Design review of the part built by this model. Coordinates are the model's own, in mm. Face numbers are marked on the shaded views. A direction names the side the tool comes from. Coordinates: 2 decimals unless noted, no trailing zeros. Write each loop counter-clockwise with the first axis right and the second up, starting at its lowest first coordinate (ties: lowest second). Pieces come first, ordered by that corner, then holes. Notation, with made-up numbers: (-4.5, 16.5) -> (27.5, 16.5) arc R18 cw to (27.5, 48.5) -> close; hole circle Ø5 at (38, -36). An arc over 180 degrees is marked (long way). One line per question, with ' | ' between items. Start each with the question number.
Q1. Add section C-C on y = -45.5. State the section outline as (x, z) points, and give its area (3 significant figures).
Q2. For P1, Ø2, axis at x = -4, z = -21.5, coming from the -Y side; P2, Ø4, axis at x = -4, y = -69.5, coming from the +Z side; P3, Ø3, axis at x = 0, y = -31.75, coming from the +Z side; P4, Ø2, axis at x = 3, z = -7.5, coming from the +Y side, all flat-tipped, find the tip position at first contact; note any pin that passes through.
Q3. Add section B-B on x = 0. Give the number of separate pieces and of enclosed holes in the cut face, and give its area (3 significant figures).
Q4. Wall thickness on probe 1 along Z at (x, y) = (3.25, -50.5); probe 2 along Z at (x, y) = (-5.5, -60.5); probe 3 along Y at (x, z) = (-0.5, -16.5): over which ranges is each line inside the solid? List them lowest first.
Q5. Add section A-A on y = -15. State the section outline as (x, z) points.
Q6. Add section D-D on y = -57.5. State the section outline as (x, z) points, and give its area (3 significant figures).
Q7. For the marked faces 5 and 6, list the 3-axis set-ups (+Z, -Z, +X, -X, +Y, -Y) from which the entire face can be reached by the end or side of a thin tool; tool diameter is ignored.
Q8. Draft analysis for pull direction Z (two halves, no side actions). For the marked faces 1, 2, 3 and 4, state which applies: pulls with the +Z half, pulls with the -Z half, needs draft (parallel to the pull), parting line crosses it, or undercut.
from build123d import *

# Parameters (mm, degrees)
BASE_FLANGE1_DEPTH     = 6.35
F_10_CLEARANCE_HOLE1_D = 5.1054
FILLET1_R              = 2.54


# Sheet-metal steps are written as plain solids
with BuildPart() as part:
    # Sketch1 → Base-Flange1 (new, symmetric)
    with BuildSketch(Plane(origin=(0, 0, 0), x_dir=(0, 0, -1), z_dir=(1, 0, 0))):
        with BuildLine():
            Line((0, 0), (0, -50.59861822))
            ThreePointArc((0, -50.59861822), (0.012620988, -50.798398969), (0.050283273, -50.995003112))
            Line((0.050283273, -50.995003112), (5.013916363, -70.244424463))
            ThreePointArc((5.013916363, -70.244424463), (12.7, -76.2), (20.386083637, -70.244424463))
            Line((20.386083637, -70.244424463), (25.349716727, -50.995003112))
            ThreePointArc((25.349716727, -50.995003112), (25.387379012, -50.798398969), (25.4, -50.59861822))
            Line((25.4, -50.59861822), (25.4, 0))
            Line((25.4, 0), (26.9875, 0))
            Line((26.9875, 0), (26.9875, -50.59861822))
            ThreePointArc((26.9875, -50.59861822), (26.962258024, -50.998179718), (26.886933455, -51.391388005))
            Line((26.886933455, -51.391388005), (21.923300364, -70.640809356))
            ThreePointArc((21.923300364, -70.640809356), (12.7, -77.7875), (3.476699636, -70.640809356))
            Line((3.476699636, -70.640809356), (-1.486933455, -51.391388005))
            ThreePointArc((-1.486933455, -51.391388005), (-1.562258024, -50.998179718), (-1.5875, -50.59861822))
            Line((-1.5875, -50.59861822), (-1.5875, 0))
            Line((-1.5875, 0), (0, 0))
        make_face()
    extrude(amount=BASE_FLANGE1_DEPTH, both=True)

    # #10 Clearance Hole1 (through all)
    with Locations(Plane.XY.offset(1.5875)):
        with Locations((0, -6.35), (0, -19.05), (0, -31.75), (0, -44.45)):
            Hole(F_10_CLEARANCE_HOLE1_D / 2)

    # Fillet1
    fillet1_edges = [part.edges().sort_by_distance(p)[0] for p in [
        (-6.35, 0, 0.79375),
        (-6.35, 0, -26.19375),
        (6.35, 0, 0.79375),
        (6.35, 0, -26.19375),
    ]]
    fillet(fillet1_edges, radius=FILLET1_R)


solid = part.part
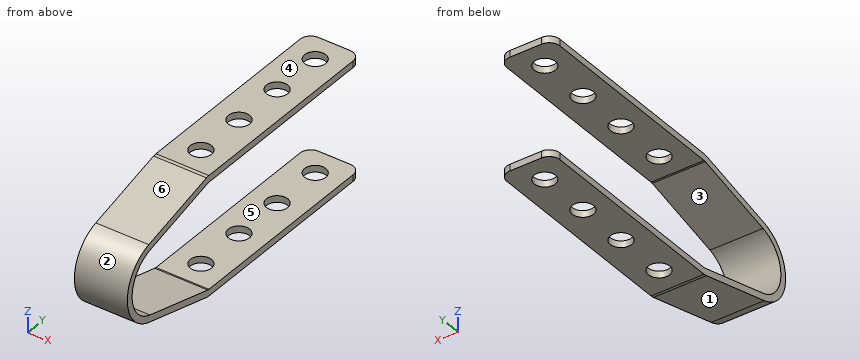
Output values:
1) outline: (-6.35, -26.99) -> (-2.33, -26.99) -> (-2.33, -25.4) -> (-6.35, -25.4) -> close; (-6.35, 0) -> (-2.33, 0) -> (-2.33, 1.59) -> (-6.35, 1.59) -> close; (2.33, -26.99) -> (6.35, -26.99) -> (6.35, -25.4) -> (2.33, -25.4) -> close; (2.33, 0) -> (6.35, 0) -> (6.35, 1.59) -> (2.33, 1.59) -> close | area: 25.5 mm2
2) P1: stops at y = -73.73 | P2: stops at z = -2.67 | P3: passes through | P4: stops at y = -73.22
3) separate pieces: 9 | enclosed holes: 0 | area: 197 mm2
4) probe 1: z = -26.99 to -25.4, 0 to 1.59 | probe 2: z = -24.54 to -22.9, -2.5 to -0.86 | probe 3: y = -77 to -75.23
5) outline: (-6.35, -26.99) -> (6.35, -26.99) -> (6.35, -25.4) -> (-6.35, -25.4) -> close; (-6.35, 0) -> (6.35, 0) -> (6.35, 1.59) -> (-6.35, 1.59) -> close
6) outline: (-6.35, -25.31) -> (6.35, -25.31) -> (6.35, -23.67) -> (-6.35, -23.67) -> close; (-6.35, -1.73) -> (6.35, -1.73) -> (6.35, -0.09) -> (-6.35, -0.09) -> close | area: 41.6 mm2
7) face 5: +X, -X, +Y | face 6: +Z, +X, -X, -Y
8) face 1: pulls with the -Z half | face 2: parting line crosses it | face 3: undercut | face 4: pulls with the +Z half
